Can you work these out from the model? Positions are in its coordinate system, mm. A direction names the side the tool comes from. Round coordinates to 2 decimals unless told otherwise and drop trailing zeros. Order: outer loops, then holes, each group sorted by start corner. A loop starts at its lowest first (then second) coordinate and runs counter-clockwise, first axis right, second up. Notation, with made-up numbers: (-38, -1.5) - (-34, -1.5) arc R7 ccw to (-34, 10.5) - close; hole circle Ø10 at (86.5, -35). An arc over 180 degrees is marked (long way). Write item = value, one per line.
from build123d import *

# Parameters (mm, degrees)
SKETCH1_W                = 60
SKETCH1_H                = 60
BOSS_EXTRUDE1_DEPTH      = 2000
BOSS_EXTRUDE2_DEPTH      = 100
BOSS_EXTRUDE2_DEPTH_BACK = 160
SKETCH2_R                = 30
BOSS_EXTRUDE3_DEPTH      = 20
BOSS_EXTRUDE3_DEPTH_BACK = 80
SKETCH3_R                = 64
SKETCH3_R_2              = 30
SKETCH4_R                = 30
CUT_EXTRUDE1_DEPTH       = 360


with BuildPart() as part:
    # Sketch1 → Boss-Extrude1 (new body)
    with BuildSketch(Plane.XY):
        with Locations((30, -30)):
            Rectangle(SKETCH1_W, SKETCH1_H)
    extrude(amount=BOSS_EXTRUDE1_DEPTH)

    # Sketch2 → Boss-Extrude2 (add, two sides: drawn at the far end of the back side and taken through both)
    with BuildSketch(Plane(origin=(0, 0, 0), x_dir=(1, 0, 0), z_dir=(0, 1, 0)).offset(-BOSS_EXTRUDE2_DEPTH_BACK)):
        with Locations(Location((30, 0, 0), (0, 0, 270))):
            Circle(SKETCH2_R)
    extrude(amount=BOSS_EXTRUDE2_DEPTH + BOSS_EXTRUDE2_DEPTH_BACK)

    # Sketch3 → Boss-Extrude3 (add, two sides: drawn at the far end of the back side and taken through both)
    with BuildSketch(Plane(origin=(60, 0, 0), x_dir=(0, 0, -1), z_dir=(1, 0, 0)).offset(-BOSS_EXTRUDE3_DEPTH_BACK)):
        with Locations(Location((-2000, -30, 0), (0, 0, 90))):
            Circle(SKETCH3_R)
        with Locations(Location((-2000, -30, 0), (0, 0, 90))):
            Circle(SKETCH3_R_2, mode=Mode.SUBTRACT)
    extrude(amount=BOSS_EXTRUDE3_DEPTH + BOSS_EXTRUDE3_DEPTH_BACK)

    # Sketch4 → Cut-Extrude1 (cut)
    with BuildSketch(Plane(origin=(80, 0, 0), x_dir=(0, 0, -1), z_dir=(1, 0, 0))):
        with Locations(Location((-2000, -30, 0), (0, 0, 90))):
            Circle(SKETCH4_R)
    extrude(amount=-CUT_EXTRUDE1_DEPTH, mode=Mode.SUBTRACT)


solid = part.part
(1) If we section it at C-C (x = 30): Write out the boundary of the cut face in (y, z), plus the area to 3 significant figures.
Computed:
outline = (-160, -30) - (100, -30) - (100, 30) - (0, 30) - (0, 1943.47) arc R64 ccw (long way) to (-60, 1943.47) - (-60, 30) - (-160, 30) - close; hole circle Ø60 at (-30, 2000)
area = 140,000 mm^2
(2) If we section it at A-A (z = 2000): Write out the boundary of the cut face in (x, y), plus the area to 3 significant figures.
Computed:
outline = (-20, -94) - (80, -94) - (80, -60) - (-20, -60) - close; (-20, 0) - (80, 0) - (80, 34) - (-20, 34) - close
area = 6,800 mm^2
(3) Thinking about a two-plate mould opening in Z: for faces 6 (the face through (30, 100, 0)), 7 (the face through (30, -60, 958)), which applies, +Z half, -Z half, draft (parallel to the pull), parting line (faces both ways), or undercut?
Computed:
face_6 = draft
face_7 = undercut
(4) If we section it at D-D (z = 427.5): Write out the boundary of the cut face in (x, y).
Computed:
outline = (0, -60) - (60, -60) - (60, 0) - (0, 0) - close
(5) If we section it at B-B (y = -30): Write out the boundary of the cut face in (x, z).
Computed:
outline = (-20, 1936) - (0, 1936) - (0, 0) arc R30 ccw to (60, 0) - (60, 1936) - (80, 1936) - (80, 1970) - (-20, 1970) - close; (-20, 2030) - (80, 2030) - (80, 2064) - (-20, 2064) - close
(6) Will these pins go through, and if not, where does the flat tip stop? P1, Ø4, axis at x = 40.5, y = 7.5, coming from the +Z side; P2, Ø18, axis at y = -32.5, z = 1323.5, coming from the -X side; P3, Ø18, axis at x = 43, z = 1099.5, coming from the -Y side.
Computed:
P1 = 2053.25
P2 = 0
P3 = -60
(7) If I drill on line 1 (Y direction, x = 41, z = 1708); line 2 (Z direction, x = 44, y = -30); line 3 (Z direction, x = -2.5, y = -45), over which ranges is the centre line in solid material (lowest first)? Write a range as from..to.
Computed:
line_1 = -60..0
line_2 = -26.53..1970, 2030..2064
line_3 = 1937.78..1974.02, 2025.98..2062.22
(8) On a 3-axis mill with a long thin cutter (end or side, diameter ignored), from which of +Z, -Z, +X, -X, +Y, -Y can I reach the whole of each face in a straight line? I mean faces 1 (the face through (0, -30, 958)), 2 (the face through (31.32, -31.82, -29.97)), 3 (the face through (80, -2, 1987)), 4 (the face through (60, -30, 958)), 5 (the face through (-20, -2, 1987)). Say none if no direction works.
Computed:
face_1 = -Z, -X, +Y, -Y
face_2 = none
face_3 = +Z, -Z, +X, +Y, -Y
face_4 = -Z, +X, +Y, -Y
face_5 = +Z, -Z, -X, +Y, -Y
